Can you work these out from the drawing? Everything is in mm from the part's minimum corner. A direction names the side the tool comes from. Round coordinates to 2 decimals unless told otherwise and drop trailing zeros. Write each loop counter-clockwise with the first axis right and the second up, starting at its lowest first coordinate (ties: lowest second). Pieces come first, ordered by that corner, then holes. Notation, with made-up numbers: (8, 67) -> (64, 67) arc R25 ccw to (64, 97) -> close; hole circle Ø4 at (59, -21). An arc over 180 degrees is marked (long way). Write item = value, one per line. Start each with the question number.
1) For the marked faces 5, 6, 7 and 8, which set-ups out of +Z, -Z, +X, -X, +Y, -Y let a thin tool reach every point of the face, with its end or its side?
2) I'm going to push flat-ended pins straight in: pin 1 (11.5 mm diameter, centred on x = 170, y = 15, fed in from +Z); pin 2 (2 mm diameter, centred on y = 26, z = 29.5, fed in from +X); pin 3 (9 mm diameter, centred on y = 17.5, z = 41.5, fed in from -X); pin 4 (8 mm diameter, centred on x = 10, y = 15, fed in from +Z). Where does each tip first touch, or does it pass through?
3) Imagine slicing it at D-D, the plane y = 5.25. Please give me the cut outline in (x, z), then the cut area to 3 significant figures.
4) If I drill on line 1 (Y direction, x = 115, z = 68.85); line 2 (X direction, y = 6.5, z = 30.5); line 3 (Z direction, x = 103, y = 23.25), over which ranges is the centre line in solid material (lowest first)?
5) Imagine slicing it at A-A, the plane x = 170. Please give me the cut outline in (y, z), then the cut area to 3 significant figures.
6) Imagine slicing it at C-C, the plane y = 15. State how many separate pieces and enclosed holes the cut face has, then the cut area to 3 significant figures.
7) Thinking about a two-plate mould opening in X: for the marked faces 1, 2, 3 and 4, which applies, +X half, -X half, draft (parallel to the pull), parting line (faces both ways), or undercut?
8) Imagine slicing it at B-B, the plane z = 9. Please give me the cut outline in (x, y), then the cut area to 3 significant figures.
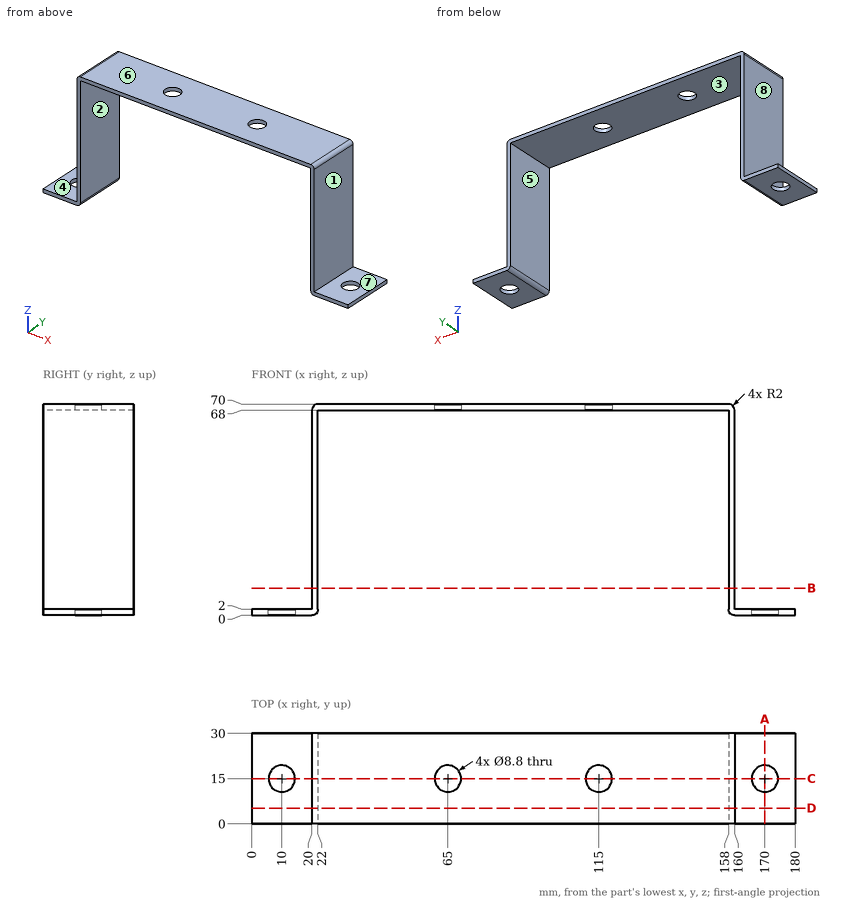
Reported:
q1.face_5 = -Z, +Y, -Y
q1.face_6 = +Z, +X, -X, +Y, -Y
q1.face_7 = +Z, +X, +Y, -Y
q1.face_8 = +Z, -X, +Y, -Y
q2.pin_1 = 2
q2.pin_2 = 160
q2.pin_3 = 20
q2.pin_4 = through
q3.outline = (0, 0) -> (20, 0) arc R2 ccw to (22, 2) -> (22, 68) -> (158, 68) -> (158, 2) arc R2 ccw to (160, 0) -> (180, 0) -> (180, 2) -> (160, 2) -> (160, 68) arc R2 ccw to (158, 70) -> (22, 70) arc R2 ccw to (20, 68) -> (20, 2) -> (0, 2) -> close
q3.area = 629 mm²
q4.line_1 = 0 to 10.6, 19.4 to 30
q4.line_2 = 20 to 22, 158 to 160
q4.line_3 = 68 to 70
q5.outline = (0, 0) -> (10.6, 0) -> (10.6, 2) -> (0, 2) -> close; (19.4, 0) -> (30, 0) -> (30, 2) -> (19.4, 2) -> close
q5.area = 42.4 mm²
q6.separate_pieces = 5
q6.enclosed_holes = 0
q6.area = 558 mm²
q7.face_1 = +X half
q7.face_2 = undercut
q7.face_3 = undercut
q7.face_4 = draft
q8.outline = (20, 0) -> (22, 0) -> (22, 30) -> (20, 30) -> close; (158, 0) -> (160, 0) -> (160, 30) -> (158, 30) -> close
q8.area = 120 mm²
